```python
from build123d import *

# Parameters (mm, degrees)
BOSS_EXTRUDE1_DEPTH = 3.175
BOSS_EXTRUDE2_DEPTH = 3.175
SKETCH3_W           = 6.236959702
SKETCH3_H           = 47.194711522
BOSS_EXTRUDE3_DEPTH = 3.175
SKETCH4_R           = 1.27
BOSS_EXTRUDE4_DEPTH = 3.175


with BuildPart() as part:
    # Sketch1 → Boss-Extrude1 (new body)
    with BuildSketch(Plane.XY):
        with BuildLine():
            Line((-17.114253333, -17.357583949), (-17.114253333, 17.357583949))
            ThreePointArc((-17.114253333, 17.357583949), (0, 24.432200125), (17.114253333, 17.357583949))
            Line((17.114253333, 17.357583949), (17.114253333, -17.357583949))
            ThreePointArc((17.114253333, -17.357583949), (0, -13.382802691), (-17.114253333, -17.357583949))
        make_face()
    extrude(amount=BOSS_EXTRUDE1_DEPTH)

    # Sketch2 → Boss-Extrude2 (add)
    with BuildSketch(Plane(origin=(0, 0, 0), x_dir=(-1, 0, 0), z_dir=(0, 0, -1))):
        with BuildLine():
            Line((-1.65128862, -13.417928303), (-1.65128862, 22.268343179))
            Line((-1.65128862, 22.268343179), (-1.65128862, 23.29835294))
            Line((-1.65128862, 23.29835294), (-2.853426735, 23.29835294))
            Line((-2.853426735, 23.29835294), (-2.853426735, -13.48778167))
            ThreePointArc((-2.853426735, -13.48778167), (-2.25262846, -13.448194961), (-1.65128862, -13.417928303))
        make_face()
        with BuildLine():
            Line((1.65128862, 23.29835294), (1.65128862, 22.268343179))
            Line((1.65128862, 22.268343179), (1.65128862, -13.417928303))
            ThreePointArc((1.65128862, -13.417928303), (2.25262846, -13.448194961), (2.853426735, -13.48778167))
            Line((2.853426735, -13.48778167), (2.853426735, 23.29835294))
            Line((2.853426735, 23.29835294), (1.65128862, 23.29835294))
        make_face()
    extrude(amount=BOSS_EXTRUDE2_DEPTH)

    # Sketch3 → Boss-Extrude3 (add)
    with BuildSketch(Plane.XY.offset(3.175)):
        with Locations((0, -23.258467244)):
            Rectangle(SKETCH3_W, SKETCH3_H)
    extrude(amount=-BOSS_EXTRUDE3_DEPTH)

    # Sketch4 → Boss-Extrude4 (add)
    with BuildSketch(Plane.XY.offset(3.175)):
        with Locations((0, -34.503683415)):
            Circle(SKETCH4_R)
    extrude(amount=BOSS_EXTRUDE4_DEPTH)


solid = part.part
```
The model under review builds one solid part; all positions refer to its coordinate system, in mm. A direction names the side the tool comes from. Round coordinates to 2 decimals unless told otherwise and drop trailing zeros. Write each loop counter-clockwise with the first axis right and the second up, starting at its lowest first coordinate (ties: lowest second). Pieces come first, ordered by that corner, then holes.
(1) We need section A-A on z = -1.25. Give the boundary of the cut face in (x, y), and give its area (3 significant figures).
(2) Wall thickness on L1, parallel to Z at x = -2, y = -24 (3 decimals); L2, parallel to X at y = -9, z = -1.25; L3, parallel to Z at x = 2.5, y = 9 (3 decimals): over which ranges is each line inside the solid? List them lowest first.
(3) We need section D-D on x = 0. Give the boundary of the cut face in (y, z) (3 decimals), and give its area (3 significant figures).
(4) We need section B-B on y = -5. Give the boundary of the cut face in (x, z) (3 decimals), and give its area (3 significant figures).
(5) We need section C-C on z = 2.5. Give the boundary of the cut face in (x, y), and give its area (3 significant figures).
(6) Mouldability with a two-part tool opening along X and no side actions: class faces 4 (the flat face through (-1.651, 5, -2)), 5 (the cylindrical face through (-0.27, 24.43, 1.57)), 6 (the flat face through (0, -46.856, 2)), 7 (the cylindrical face through (10.4, -14.8, 1.6)) as +X half, -X half, draft (parallel to the pull), parting line (faces both ways), or undercut.
(7) Machinability: for faces 1 (the cylindrical face through (-2.244, -13.448, -1.565)), 2 (the flat face through (2.853, 5, -2)), 3 (the flat face through (-2, 23.298, -2)), which of the approach directions +Z, -Z, +X, -X, +Y, -Y give a long, thin tool a straight path to every point of the face, cutting with its end or side? Answer none if there is none.
(8) Insertion check: pin 1 (1 mm diameter, centred on y = 7, z = -2, fed in from -X); pin 2 (1.6 mm diameter, centred on y = 11.5, z = -2, fed in from +X); pin 3 (1 mm diameter, centred on y = -28.5, z = 1, fed in from +X). Each pin has a flat end and moves straight along its axis. Give the tip position at first contact, or say it passes through.
Findings below:
1. outline: (-2.85, -13.49) arc R38.83 cw to (-1.65, -13.42) - (-1.65, 23.3) - (-2.85, 23.3) - close; (1.65, -13.42) arc R38.83 cw to (2.85, -13.49) - (2.85, 23.3) - (1.65, 23.3) - close
1. area: 88.4 mm2
2. L1: z = 0 to 3.175
2. L2: x = -2.85 to -1.65, 1.65 to 2.85
2. L3: z = -3.175 to 3.175
3. outline: (-46.856, 0) - (24.432, 0) - (24.432, 3.175) - (-33.234, 3.175) - (-33.234, 6.35) - (-35.774, 6.35) - (-35.774, 3.175) - (-46.856, 3.175) - close
3. area: 234 mm2
4. outline: (-17.114, 0) - (-2.853, 0) - (-2.853, -3.175) - (-1.651, -3.175) - (-1.651, 0) - (1.651, 0) - (1.651, -3.175) - (2.853, -3.175) - (2.853, 0) - (17.114, 0) - (17.114, 3.175) - (-17.114, 3.175) - close
4. area: 116 mm2
5. outline: (-17.11, -17.36) arc R38.83 cw to (-3.12, -13.51) - (-3.12, -46.86) - (3.12, -46.86) - (3.12, -13.51) arc R38.83 cw to (17.11, -17.36) - (17.11, 17.36) arc R24.24 ccw to (-17.11, 17.36) - close
5. area: 1,470 mm2
6. face 4: undercut
6. face 5: parting line
6. face 6: draft
6. face 7: undercut
7. face 1: -Z, -Y
7. face 2: -Z, +X, +Y, -Y
7. face 3: -Z, +X, -X, +Y
8. pin 1: stops at x = -2.85
8. pin 2: stops at x = 2.85
8. pin 3: stops at x = 3.12
